Print and shaded views of the part. All mm, measured from the part's lowest x, y and z. A direction names the side the tool comes from. Round coordinates to 2 decimals unless told otherwise and drop trailing zeros. Write each loop counter-clockwise with the first axis right and the second up, starting at its lowest first coordinate (ties: lowest second). Pieces come first, ordered by that corner, then holes. Notation, with made-up numbers: (-28.75, -9) - (9.25, -9) arc R27 cw to (9.25, 22) - close; hole circle Ø4 at (89.25, 39.5). An arc over 180 degrees is marked (long way). One line per item, written item: value.
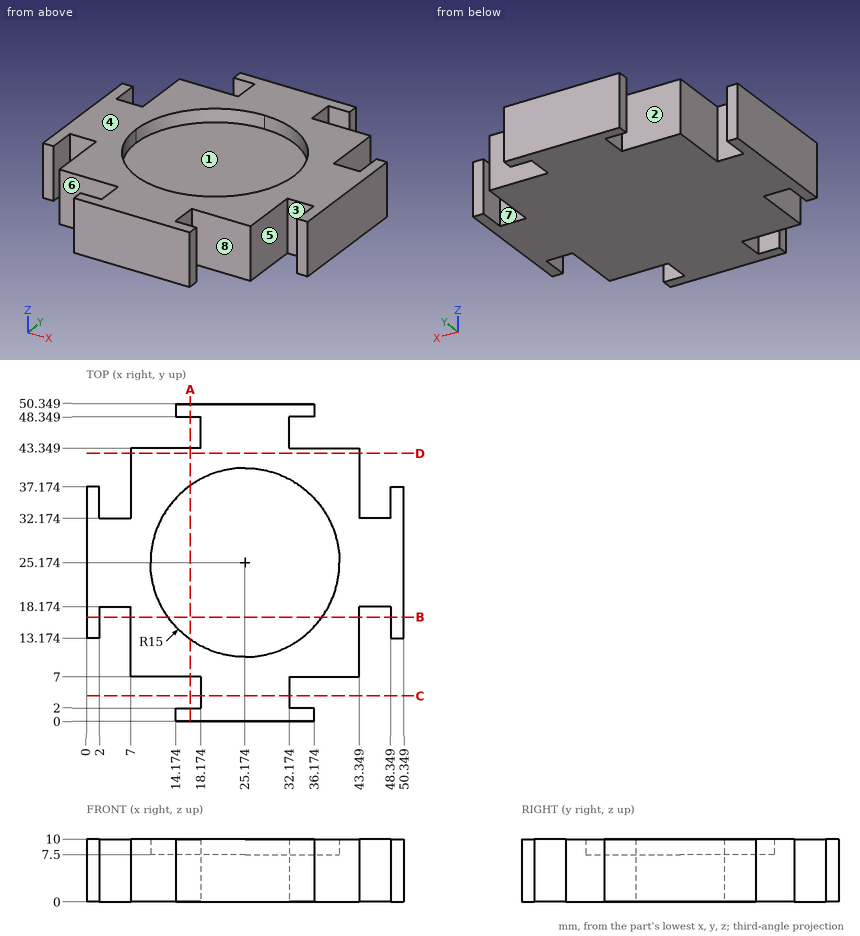
1. Band-saw the part on C-C on y = 4. Write the cut outline in (x, z) (1 decimal).
Report:
outline: (18.2, 0) - (32.2, 0) - (32.2, 10) - (18.2, 10) - close
2. Drop flat-ended pins along their axis: pin 1 (2.5 mm diameter, centred on x = 4.5, z = 5, fed in from -Y); pin 2 (4 mm diameter, centred on y = 47, z = 7, fed in from -X); pin 3 (2 mm diameter, centred on x = 1, z = 6, fed in from -Y). Give the stop position or say it passes through.
Report:
pin 1: y = 18.17
pin 2: x = 14.17
pin 3: y = 13.17
3. Mould opens along Y. For the marked faces 1, 2, 3 and 4 say: released by +Y, released by -Y, zero draft, split by the parting line, or undercut.
Report:
face 1: undercut
face 2: undercut
face 3: released by -Y
face 4: zero draft
4. Band-saw the part on A-A on x = 16.5. Write the cut outline in (y, z).
Report:
outline: (0, 0) - (2, 0) - (2, 10) - (0, 10) - close; (7, 0) - (43.35, 0) - (43.35, 10) - (37.41, 10) - (37.41, 7.5) - (12.94, 7.5) - (12.94, 10) - (7, 10) - close; (48.35, 0) - (50.35, 0) - (50.35, 10) - (48.35, 10) - close
5. Band-saw the part on D-D on y = 42.5. Write the cut outline in (x, z).
Report:
outline: (7, 0) - (43.35, 0) - (43.35, 10) - (7, 10) - close
6. Wall check: probe 1 along X at (y, z) = (36, 4.25); probe 2 along X at (y, z) = (42, 2.75). Give the ranges that are in metal, low to high. Write a range as [from, to].
Report:
probe 1: [0, 2], [7, 43.35], [48.35, 50.35]
probe 2: [7, 43.35]
7. Tool access for the marked faces 5, 6, 7 and 8: list every direction of +Z, -Z, +X, -X, +Y, -Y with a clear straight run to the whole face (end or side of a thin tool).
Report:
face 5: +Z, -Z, -Y
face 6: +Z, -Z, -X
face 7: +Z, -Z, +Y
face 8: +Z, -Z, +X
